```python
from build123d import *

# Parameters (mm, degrees)
F0_R     = 7.9375
F1_DEPTH = 361.95
F0_R_2   = 9.525
F2_DEPTH = 349.25
F3_DEPTH = 76.2
F5_W     = 5.461208
F5_H     = 50.8
F6_DEPTH = 4.7625
F8_W     = 25.4
F8_H     = 25.4
F9_DEPTH = 2.54


with BuildPart() as f1:
    # F0 (on Top) → F1 (new body)
    with BuildSketch(Plane.XY):
        Circle(F0_R)
    extrude(amount=F1_DEPTH)

    # F0 (on Top) → F2 (join)
    with BuildSketch(Plane.XY):
        Circle(F0_R_2)
        Circle(F0_R, mode=Mode.SUBTRACT)
    extrude(amount=F2_DEPTH)

    # F0 (on Top) → F3 (cut)
    with BuildSketch(Plane.XY):
        Circle(F0_R_2)
        Circle(F0_R, mode=Mode.SUBTRACT)
    extrude(amount=F3_DEPTH, mode=Mode.SUBTRACT)

    # F5 (on offset) → F6 (cut)
    with BuildSketch(Plane.YZ.offset(7.9375)):
        with Locations((0, 25.4)):
            Rectangle(F5_W, F5_H)
    extrude(amount=-F6_DEPTH, mode=Mode.SUBTRACT)

    # F8 (on offset) → F9 (cut)
    with BuildSketch(Plane.YZ.offset(9.525)):
        with Locations((0, 309.224188)):
            Rectangle(F8_W, F8_H)
        with Locations((0, 106.897242)):
            Rectangle(F8_W, F8_H)
    extrude(amount=-F9_DEPTH, mode=Mode.SUBTRACT)


solid = f1.part
```
The model under review builds one solid part; all positions refer to its coordinate system, in mm. A direction names the side the tool comes from. Give positions to 0.01 mm unless a question says otherwise; leave off trailing zeros. Write each loop counter-clockwise with the first axis right and the second up, starting at its lowest first coordinate (ties: lowest second). Pieces come first, ordered by that corner, then holes. Notation, with made-up numbers: (-21.75, -38.75) - (9.25, -38.75) arc R29 cw to (9.25, -8.75) - close; hole circle Ø7 at (62.5, 41.5). An arc over 180 degrees is marked (long way). Answer in a Markdown table with one row per item. Add a question column.
1. Wall thickness on line 1 along Z through (x, y) = (-7.75, 4); line 2 along X through (y, z) = (-7, 336); line 3 along Y through (x, z) = (-7.75, 221): over which ranges is each line inside the solid? List them lowest first. Write a range as [from, to].
2. Tool access review of faces 1 (the cylindrical face through (-1.72, -7.75, 355.51)), 2 (the flat face through (0, 0, 361.95)), 3 (the cylindrical face through (-6.3, -4.83, 37.57)): name each direction out of +Z, -Z, +X, -X, +Y, -Y from which nothing blocks a thin tool from reaching the whole face with its end or side.
3. We need section B-B on z = 140.5. Write out the cut boundary in (x, y) (3 decimals), then the cut area to 3 significant figures.
4. We need section A-A on x = -4. Write out the cut boundary in (y, z).
5. We need section C-C on z = 47. Write out the cut boundary in (x, y) (1 decimal), then the cut area to 3 significant figures.
6. Insertion check: P1, Ø8, axis at x = 5, z = 221.5, coming from the -Y side; P2, Ø1.3, axis at x = 8.5, y = -0.5, coming from the -Z side; P3, Ø1.5, axis at y = 3.5, z = 255, coming from the +X side. Each pin has a flat end and moves straight along its axis. Give the tip position at first contact, or say it passes through.
7. Draft analysis for pull direction Z (two halves, no side actions). For faces 4 (the flat face through (0, 0, 0)), 5 (the flat face through (6.985, 0, 309)), 6 (the flat face through (3.175, 0, 26)), 7 (the flat face through (6.985, 0, 107)), state which applies: +Z half, -Z half, draft (parallel to the pull), parting line (faces both ways), or undercut.
Ans:
| question | item | result |
|---|---|---|
| 1 | line 1 | z = [76.2, 349.25] |
| 1 | line 2 | x = [-6.46, 6.46] |
| 1 | line 3 | y = [-5.54, 5.54] |
| 2 | face 1 | +Z |
| 2 | face 2 | +Z, +X, -X, +Y, -Y |
| 2 | face 3 | -Z |
| 3 | outline | circle Ø19.05 at (0, 0) |
| 3 | area | 285 mm^2 |
| 4 | outline | (-8.64, 76.2) - (-6.86, 76.2) - (-6.86, 0) - (6.86, 0) - (6.86, 76.2) - (8.64, 76.2) - (8.64, 349.25) - (6.86, 349.25) - (6.86, 361.95) - (-6.86, 361.95) - (-6.86, 349.25) - (-8.64, 349.25) - close |
| 5 | outline | (3.2, -2.7) - (3.2, 2.7) - (7.5, 2.7) arc R7.9 ccw (long way) to (7.5, -2.7) - close |
| 5 | area | 173 mm^2 |
| 6 | P1 | stops at y = -9.47 |
| 6 | P2 | stops at z = 50.8 |
| 6 | P3 | stops at x = 9.12 |
| 7 | face 4 | -Z half |
| 7 | face 5 | undercut |
| 7 | face 6 | draft |
| 7 | face 7 | undercut |
